Design review of the part built by this model. Coordinates are the model's own, in mm. Coordinates: 2 decimals unless noted, no trailing zeros. Loops run counter-clockwise (first coordinate to the right, second up) from the corner with the lowest first, then second, coordinate; pieces in that order, holes last. Notation, with made-up numbers: (77.5, 27.5) -> (99.5, 27.5) arc R24 cw to (99.5, 56.5) -> close; hole circle Ø7 at (50, 0). An arc over 180 degrees is marked (long way). Use CSV: the item, a comma, the result in double quotes.
```python
from build123d import *

# Parameters (mm, degrees)
SKETCH1_W           = 175
SKETCH1_H           = 70
BOSS_EXTRUDE1_DEPTH = 3
SKETCH2_W           = 20
SKETCH2_H           = 25
CUT_EXTRUDE1_DEPTH  = 5
FILLET1_R           = 4
FILLET2_R           = 15


with BuildPart() as part:
    # Sketch1 → Boss-Extrude1 (new body)
    with BuildSketch(Plane(origin=(0, 0, 0), x_dir=(1, 0, 0), z_dir=(0, 1, 0))):
        with Locations((87.5, 35)):
            Rectangle(SKETCH1_W, SKETCH1_H)
    extrude(amount=BOSS_EXTRUDE1_DEPTH)

    # Sketch2 → Cut-Extrude1 (cut)
    with BuildSketch(Plane(origin=(0, 3, 0), x_dir=(1, 0, 0), z_dir=(0, 1, 0))):
        with Locations((87.5, 12.5)):
            Rectangle(SKETCH2_W, SKETCH2_H)
        with BuildLine():
            Line((11, 10), (11, 0))
            Line((11, 0), (4, 0))
            Line((4, 0), (4, 10))
            ThreePointArc((4, 10), (7.5, 13.5), (11, 10))
        make_face()
        with BuildLine():
            Line((171, 0), (171, 10))
            ThreePointArc((171, 10), (167.5, 13.5), (164, 10))
            Line((164, 10), (164, 0))
            Line((164, 0), (171, 0))
        make_face()
    extrude(amount=-CUT_EXTRUDE1_DEPTH, mode=Mode.SUBTRACT)

    # Fillet1
    fillet1_edges = [part.edges().sort_by_distance(p)[0] for p in [
        (77.5, 1.5, -25),
        (97.5, 1.5, -25),
    ]]
    fillet(fillet1_edges, radius=FILLET1_R)

    # Fillet2
    fillet2_edges = [part.edges().sort_by_distance(p)[0] for p in [
        (0, 1.5, -70),
        (175, 1.5, -70),
    ]]
    fillet(fillet2_edges, radius=FILLET2_R)


solid = part.part
```
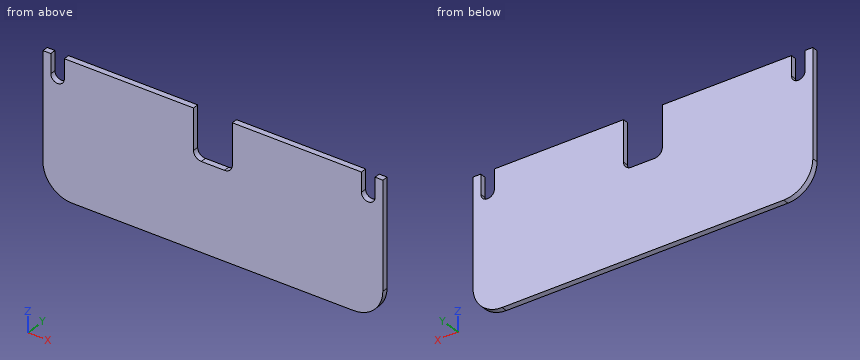
Item 1: Clearance check with flat-ended pins moving along their axes: pin 1 (1 mm diameter, centred on x = 128.5, y = 1, fed in from +Z); pin 2 (1.5 mm diameter, centred on x = 87, y = 1.5, fed in from +Z). State where each tip first meets the part, or that it passes through.
Checked values:
pin 1,"z = 0"
pin 2,"z = -25"
Item 2: Add section B-B (y = 0.8). Give the boundary of the cut face in (x, z).
Checked values:
outline,"(0, -55) arc R15 ccw to (15, -70) -> (160, -70) arc R15 ccw to (175, -55) -> (175, 0) -> (171, 0) -> (171, -10) arc R3.5 cw to (164, -10) -> (164, 0) -> (97.5, 0) -> (97.5, -21) arc R4 cw to (93.5, -25) -> (81.5, -25) arc R4 cw to (77.5, -21) -> (77.5, 0) -> (11, 0) -> (11, -10) arc R3.5 cw to (4, -10) -> (4, 0) -> (0, 0) -> close"
Item 3: Add section D-D (z = -62). Give the boundary of the cut face in (x, y), then the cut area to 3 significant figures.
Checked values:
outline,"(1.73, 0) -> (173.27, 0) -> (173.27, 3) -> (1.73, 3) -> close"
area,"515 mm^2"
Item 4: Add section A-A (z = -4.5). Give the boundary of the cut face in (x, y), then the cut area to 3 significant figures.
Checked values:
outline,"(0, 0) -> (4, 0) -> (4, 3) -> (0, 3) -> close; (11, 0) -> (77.5, 0) -> (77.5, 3) -> (11, 3) -> close; (97.5, 0) -> (164, 0) -> (164, 3) -> (97.5, 3) -> close; (171, 0) -> (175, 0) -> (175, 3) -> (171, 3) -> close"
area,"423 mm^2"
Item 5: Add section C-C (x = 167.5). Give the boundary of the cut face in (y, z).
Checked values:
outline,"(0, -67.99) -> (3, -67.99) -> (3, -13.5) -> (0, -13.5) -> close"
Item 6: To check wall thickness, follow line 1 along X through (y, z) = (2.05, -8); line 2 along Z through (x, y) = (12, 1.5); line 3 along Z through (x, y) = (13, 2). State the ranges of each line that lie inside material, in increasing order.
Checked values:
line 1,"0 to 4, 11 to 77.5, 97.5 to 164, 171 to 175"
line 2,"-69.7 to 0"
line 3,"-69.87 to 0"
